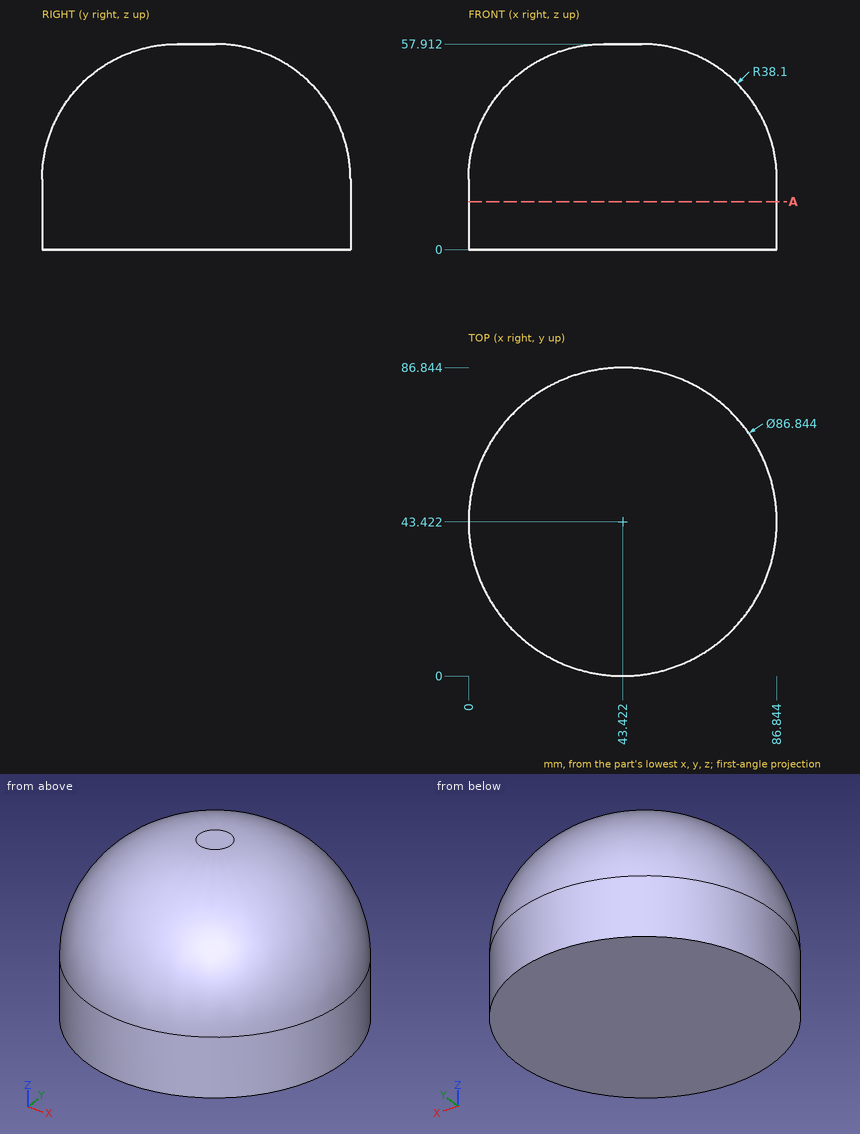
Job drawing, mm, ordinate dimensions from the low corner. One solid piece. Round coordinates to 2 decimals unless told otherwise and drop trailing zeros. Order: outer loops, then holes, each group sorted by start corner. A loop starts at its lowest first (then second) coordinate and runs counter-clockwise, first axis right, second up. Notation, with made-up numbers: M 71.5,-27 L 75.5,-27 A29 cw 75.5,7 Z; hole C 40,36 d5. An arc over 180 degrees is marked long. Write each question's results on one line, items separated by ' | '. Start each with the question number.
(1) Probe probe 1 along Y at (x, z) = (56, 41.5); probe 2 along Y at (x, z) = (29, 8) (1 decimal); probe 3 along X at (y, z) = (64.5, 22.5). List the from-to ranges inside material, lowest first. Write a range as from..to.
(2) Drop flat-ended pins along their axis: pin 1 (8 mm diameter, centred on x = 62, z = 8.5, fed in from -Y); pin 2 (6 mm diameter, centred on y = 36.5, z = 42, fed in from -X); pin 3 (5 mm diameter, centred on x = 47, y = 73, fed in from +Z). Give the stop position or say it passes through.
(3) Saw through at A-A, the plane z = 13.5. Give the cut face in (x, y).
Established:
1) probe 1: y = 9..77.84 | probe 2: y = 2.5..84.4 | probe 3: x = 5.57..81.28
2) pin 1: stops at y = 2.52 | pin 2: stops at x = 5.74 | pin 3: stops at z = 50.94
3) outline: C 43.42,43.42 d86.84
